Model file for the job. Use its own axes, mm. A direction names the side the tool comes from. Coordinates: 2 decimals unless noted, no trailing zeros. Write each loop counter-clockwise with the first axis right and the second up, starting at its lowest first coordinate (ties: lowest second). Pieces come first, ordered by that corner, then holes.
Q1. Pin check, flat tips, straight feed: P1, Ø4, axis at y = 2.5, z = -10.5, coming from the +X side; P2, Ø3, axis at x = 5.5, z = 7, coming from the +Y side; P3, Ø3, axis at x = 0.5, z = 39.5, coming from the +Y side. Stop position of each tip, or through.
Q2. Drill centre lines: probe 1 along Z at (x, y) = (5, -11); probe 2 along X at (y, z) = (-1.5, -7); probe 3 along X at (y, z) = (6, 35.5). Where is each one in solid material? Low to high.
Q3. Band-saw the part on B-B, the plane x = 1. Write the cut outline in (y, z), plus the area to 3 significant figures.
Q4. Band-saw the part on C-C, the plane z = 45. Write the cut outline in (x, y).
Q5. Band-saw the part on A-A, the plane y = 0. Write the cut outline in (x, z).
Q6. Pull direction Y, two halves, no side cores. Call faces 4 (the cylindrical face through (-3.47, -15.62, 3.94)), 5 (the flat face through (-3.8, 7.3, 8)): released by +Y, released by -Y, zero draft, split by the parting line, or undercut.
Q7. Which spindle directions (+Z, -Z, +X, -X, +Y, -Y) get a long thin tool onto all of the face, cutting with end or side? Do faces 1 (the cylindrical face through (-1.73, -7.81, 32.65)), 2 (the flat face through (0, 0, -34)), 3 (the cylindrical face through (-1.73, 7.81, -17.24)). Say none if no direction does.
Q8. Band-saw the part on D-D, the plane z = 1.5. Write the cut outline in (x, y).
from build123d import *

# Parameters (mm, degrees)
ESQUISSE1_R          = 16
BASE_EXTRUSION_DEPTH = 8
ESQUISSE2_R          = 8
BOSS_EXTRU_1_DEPTH   = 50
BOSS_EXTRU_2_START   = 34
ESQUISSE3_R          = 8
BOSS_EXTRU_2_DEPTH   = 34


with BuildPart() as part:
    # Esquisse1 → Base-Extrusion (new body)
    with BuildSketch(Plane.XY):
        Circle(ESQUISSE1_R)
    extrude(amount=BASE_EXTRUSION_DEPTH)

    # Esquisse2 → Boss.-Extru.1 (add)
    with BuildSketch(Plane.XY.offset(8)):
        Circle(ESQUISSE2_R)
    extrude(amount=BOSS_EXTRU_1_DEPTH)

    # Esquisse3 → Boss.-Extru.2 (add)
    with BuildSketch(Plane(origin=(0, 0, 0), x_dir=(-1, 0, 0), z_dir=(0, 0, -1)).offset(BOSS_EXTRU_2_START)):
        with Locations(Location((0, 0, 0), (0, 0, 180))):
            Circle(ESQUISSE3_R)
    extrude(amount=-BOSS_EXTRU_2_DEPTH)


solid = part.part
Answer sheet:
1. P1: stops at x = 7.98
1. P2: stops at y = 15.49
1. P3: stops at y = 8
2. probe 1: z = 0 to 8
2. probe 2: x = -7.86 to 7.86
2. probe 3: x = -5.29 to 5.29
3. outline: (-15.97, 0) - (-7.94, 0) - (-7.94, -34) - (7.94, -34) - (7.94, 0) - (15.97, 0) - (15.97, 8) - (7.94, 8) - (7.94, 58) - (-7.94, 58) - (-7.94, 8) - (-15.97, 8) - close
3. area: 1,590 mm2
4. outline: circle Ø16 at (0, 0)
5. outline: (-16, 0) - (-8, 0) - (-8, -34) - (8, -34) - (8, 0) - (16, 0) - (16, 8) - (8, 8) - (8, 58) - (-8, 58) - (-8, 8) - (-16, 8) - close
6. face 4: split by the parting line
6. face 5: zero draft
7. face 1: +Z
7. face 2: -Z, +X, -X, +Y, -Y
7. face 3: -Z
8. outline: circle Ø32 at (0, 0)
